Read the model definition and answer for the solid it produces. Units are mm, in the model's axes. Face numbers are marked on the shaded views. A direction names the side the tool comes from. Coordinates: 2 decimals unless noted, no trailing zeros. Write item = value, one per line.
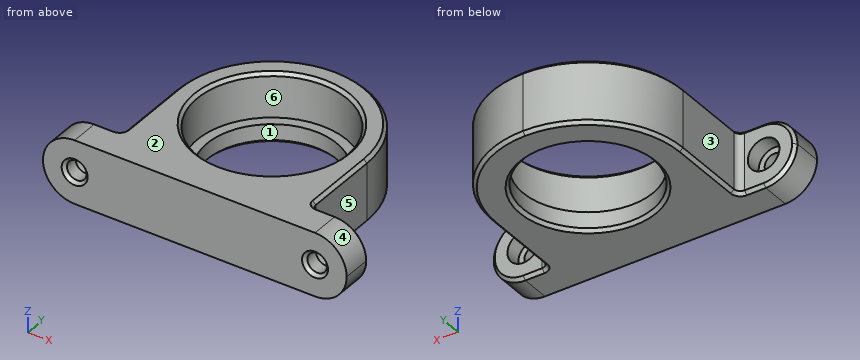
from build123d import *

# Parameters (mm, degrees)
SKETCH_1_W          = 96
SKETCH_1_H          = 20
EXTRUDE_1_DEPTH     = 10
SKETCH_2_R          = 5
CUT_EXTRUDE_1_DEPTH = 5
FILLET_1_R          = 10
SKETCH_3_R          = 3.1
CUT_EXTRUDE_2_DEPTH = 5
CHAMFER_1_SIZE      = 1
SKETCH_4_W          = 60
SKETCH_4_H          = 20
EXTRUDE_2_DEPTH     = 55.5
CUT_EXTRUDE_START   = -20
CUT_EXTRUDE_3_DEPTH = 20
SKETCH_6_4_R        = 23.6
CUT_EXTRUDE_4_DEPTH = 14
SKETCH_7_R          = 20.5
CUT_EXTRUDE_5_DEPTH = 10
FILLET_2_R          = 2
CHAMFER_2_SIZE      = 1
CHAMFER_3_SIZE      = 1


# Read off the part's stored shape, not the designer's step: 切除-拉伸3
with BuildPart() as part:
    # 草图1 → 凸台-拉伸1 (new body)
    with BuildSketch(Plane(origin=(0, 0, 0), x_dir=(1, 0, 0), z_dir=(0, 1, 0))):
        Rectangle(SKETCH_1_W, SKETCH_1_H)
    extrude(amount=EXTRUDE_1_DEPTH)

    # 草图2 → 切除-拉伸1 (cut)
    with BuildSketch(Plane(origin=(0, 10, 0), x_dir=(1, 0, 0), z_dir=(0, 1, 0))):
        with Locations(Location((-38, 0, 0), (0, 0, 270))):
            Circle(SKETCH_2_R)
        with Locations(Location((38, 0, 0), (0, 0, 90))):
            Circle(SKETCH_2_R)
    extrude(amount=-CUT_EXTRUDE_1_DEPTH, mode=Mode.SUBTRACT)

    # 圆角1
    fillet_1_edges = [part.edges().sort_by_distance(p)[0] for p in [
        (48, 5, -10),
        (48, 5, 10),
        (-48, 5, 10),
        (-48, 5, -10),
    ]]
    fillet(fillet_1_edges, radius=FILLET_1_R - 0.0001)  # a hair under: the kernel refuses the full size

    # 草图3 → 切除-拉伸2 (cut)
    with BuildSketch(Plane(origin=(0, 5, 0), x_dir=(1, 0, 0), z_dir=(0, 1, 0))):
        with Locations(Location((-38, 0, 0), (0, 0, 270))):
            Circle(SKETCH_3_R)
        with Locations(Location((38, 0, 0), (0, 0, 270))):
            Circle(SKETCH_3_R)
    extrude(amount=-CUT_EXTRUDE_2_DEPTH, mode=Mode.SUBTRACT)

    # 倒角1
    chamfer_1_edges = [part.edges().sort_by_distance(p)[0] for p in [
        (-38, 0, -3.1),
        (38, 0, -3.1),
    ]]
    chamfer(chamfer_1_edges, length=CHAMFER_1_SIZE)

    # 草图4 → 凸台-拉伸2 (add)
    with BuildSketch(Plane(origin=(0, 10, 0), x_dir=(1, 0, 0), z_dir=(0, 1, 0))):
        Rectangle(SKETCH_4_W, SKETCH_4_H)
    extrude(amount=EXTRUDE_2_DEPTH)

    # 切除-拉伸3 outline → 切除-拉伸3 (cut)
    with BuildSketch(Plane.XY.offset(10).offset(CUT_EXTRUDE_START)):
        with BuildLine():
            Line((-30, 65.5), (-30, 35.5))
            ThreePointArc((-30, 35.5), (-21.213203436, 56.713203436), (0, 65.5))
            Line((0, 65.5), (-30, 65.5))
        make_face()
        with BuildLine():
            Line((30, 65.5), (0, 65.5))
            ThreePointArc((0, 65.5), (21.213203436, 56.713203436), (30, 35.5))
            Line((30, 35.5), (30, 65.5))
        make_face()
    extrude(amount=CUT_EXTRUDE_3_DEPTH, mode=Mode.SUBTRACT)

    # 草图6<4> → 切除-拉伸4 (cut)
    with BuildSketch(Plane.XY.offset(10)):
        with Locations((0, 35.5)):
            Circle(SKETCH_6_4_R)
    extrude(amount=-CUT_EXTRUDE_4_DEPTH, mode=Mode.SUBTRACT)

    # 草图7 → 切除-拉伸5 (cut)
    with BuildSketch(Plane.XY.offset(-4)):
        with Locations((0, 35.5)):
            Circle(SKETCH_7_R)
    extrude(amount=-CUT_EXTRUDE_5_DEPTH, mode=Mode.SUBTRACT)

    # 圆角2
    fillet_2_edges = [part.edges().sort_by_distance(p)[0] for p in [
        (30, 10, 0),
        (-30, 10, 0),
    ]]
    fillet(fillet_2_edges, radius=FILLET_2_R)

    # 倒角2
    chamfer_2_edges = [part.edges().sort_by_distance(p)[0] for p in [
        (35.00005, 10, 10),
        (35.00005, 10, -10),
        (30.585786438, 10.585786438, -10),
        (30.585786438, 10.585786438, 10),
        (-30.585786438, 10.585786438, 10),
        (-30.585786438, 10.585786438, -10),
        (-35.00005, 10, -10),
        (-35.00005, 10, 10),
        (-45.071097101, 10, -7.071097101),
        (-45.071097101, 10, 7.071097101),
        (45.071097101, 10, 7.071097101),
        (45.071097101, 10, -7.071097101),
        (-30, 23.75, 10),
        (-30, 23.75, -10),
        (30, 23.75, -10),
        (30, 23.75, 10),
        (21.213203436, 56.713203436, -10),
        (-21.213203436, 56.713203436, 10),
    ]]
    chamfer(chamfer_2_edges, length=CHAMFER_2_SIZE)

    # 倒角3
    chamfer_3_edges = [part.edges().sort_by_distance(p)[0] for p in [
        (-20.5, 35.5, -10),
        (-23.6, 35.5, 10),
    ]]
    chamfer(chamfer_3_edges, length=CHAMFER_3_SIZE)


solid = part.part
1) Flat-ended cylindrical pins translate along their axes: pin 1 Ø9 at (x, z) = (-38, 0) entering from +Y; pin 2 Ø5.5 at (x, z) = (-38, 0) entering from -Y; pin 3 Ø8 at (x, z) = (39, -1.5) entering from +Y; pin 4 Ø4 at (y, z) = (56.5, 0) entering from -X. Find the tip coordinate at first contact, or state that the pin passes through.
Returned:
pin_1 = 5
pin_2 = through
pin_3 = 10
pin_4 = -23.22
2) Determine the mould class of the marked faces 1, 2 and 3 for opening direction X: pulls with the +X half, pulls with the -X half, needs draft (parallel to the pull), parting line crosses it, or undercut.
Returned:
face_1 = undercut
face_2 = needs draft
face_3 = pulls with the -X half
3) The part is cut by section A-A (z = 2). Count the separate pieces of the cut face and the enclosed holes in it, and give its area (3 significant figures).
Returned:
separate_pieces = 3
enclosed_holes = 1
area = 2,010 mm^2
4) Straight lines are drawn through the part: line 1 along X through (y, z) = (7.8, 0); line 2 along X through (y, z) = (1.9, 0); line 3 along Y through (x, z) = (0, 2). For each, find the intervals that lie inside material, in ascending order. Write a range as from..to.
Returned:
line_1 = -48..-43, -33..33, 43..48
line_2 = -48..-41.1, -34.9..34.9, 41.1..48
line_3 = 0..11.9, 59.1..65.5
5) For the marked faces 4, 5 and 6, determine the directions among +Z, -Z, +X, -X, +Y, -Y from which every point of the face is accessible in a straight line to the end or side of a thin tool.
Returned:
face_4 = +Z, +X, +Y, -Y
face_5 = +Z, -Z, +X, +Y
face_6 = +Z
